Part model, mm, in its own coordinate system. Face numbers are marked on the shaded views. A direction names the side the tool comes from. Round coordinates to 2 decimals unless told otherwise and drop trailing zeros. Write each loop counter-clockwise with the first axis right and the second up, starting at its lowest first coordinate (ties: lowest second). Pieces come first, ordered by that corner, then holes. Notation, with made-up numbers: (19, 34.25) -> (37, 34.25) arc R7 ccw to (37, 38.25) -> close; hole circle Ø8 at (53, 73.5). An arc over 180 degrees is marked (long way). Use CSV: the item, a comma, the result in double quotes. Start each with the question number.
```python
from build123d import *

# Parameters (mm, degrees)
F1_DEPTH = 63.5
F2_DEPTH = 7.9375
F3_DEPTH = 25.4
F5_R     = 6.35


with BuildPart() as f1:
    # F0 (on Front) → F1 (new body, symmetric)
    with BuildSketch(Plane.XZ):
        Polygon((-41.275, 9.525), (-41.275, -9.525), (41.275, -9.525), (41.275, 9.525), (22.225, 9.525), align=None)
    extrude(amount=F1_DEPTH, both=True)

    # F0 (on Front) → F2 (join, symmetric)
    with BuildSketch(Plane.XZ):
        with BuildLine():
            add(Edge.make_bspline(
                [(-41.275, 9.525), (-40.209185, 45.154918), (21.977982, 81.660934), (57.15, 80.9752)],
                knots=[0, 0, 0, 0, 121.624881, 121.624881, 121.624881, 121.624881], degree=3))
            Line((-41.275, 9.525), (22.225, 9.525))
            Line((22.225, 9.525), (22.225, 46.0502))
            ThreePointArc((22.225, 46.0502), (32.454296, 70.745904), (57.15, 80.9752))
        make_face()
    extrude(amount=F2_DEPTH, both=True)

    # F0 (on Front) → F3 (join, symmetric)
    with BuildSketch(Plane.XZ):
        with BuildLine():
            Line((22.225, 9.525), (41.275, 9.525))
            Line((41.275, 9.525), (41.275, 46.0502))
            ThreePointArc((41.275, 46.0502), (45.92468, 57.27552), (57.15, 61.9252))
            Line((57.15, 61.9252), (60.325, 61.9252))
            Line((60.325, 61.9252), (60.325, 80.9752))
            Line((60.325, 80.9752), (57.15, 80.9752))
            ThreePointArc((57.15, 80.9752), (32.454296, 70.745904), (22.225, 46.0502))
            Line((22.225, 46.0502), (22.225, 9.525))
        make_face()
    extrude(amount=F3_DEPTH, both=True)

    # F0 (on Front) → F4 (revolve)
    with BuildSketch(Plane.XZ):
        Polygon((60.325, 85.725), (60.325, 80.9752), (85.754924, 80.9752), (85.754924, 61.9252), (60.325, 61.9252), (60.325, 57.15), (111.125, 57.15), (111.125, 85.725), align=None)
    revolve(axis=Axis((60.325, 0, 71.4375), (0, 0, -1)))

    # F5
    f5_edges = [f1.edges().sort_by_distance(p)[0] for p in [
        (41.275, -63.5, 0),
        (-41.275, -63.5, 0),
        (41.275, 63.5, 0),
        (-41.275, 63.5, 0),
    ]]
    fillet(f5_edges, radius=F5_R)


solid = f1.part
```
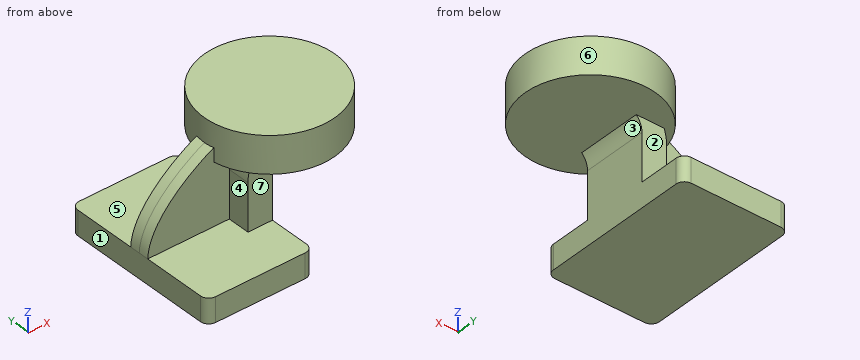
1. Band-saw the part on B-B (z = -3.5). List the corners of the cut face in (x, y) (3 decimals), then the cut area to 3 significant figures.
2. Pull direction Z, two halves, no side cores. Call the marked faces 1, 2 and 3: released by +Z, released by -Z, zero draft, split by the parting line, or undercut.
3. Drill centre lines: line 1 along Z through (x, y) = (74.5, 21) (3 decimals); line 2 along Y through (x, z) = (-19.5, 10); line 3 along Z through (x, y) = (87.5, 3) (3 decimals). Where is each one in solid material? Low to high. Write a range as [from, to].
4. Band-saw the part on D-D (y = -11). List the corners of the cut face in (x, z) (3 decimals).
5. Flat gauge pins, fed straight in: pin 1 (12 mm diameter, centred on x = 11.5, y = 44.5, fed in from +Z) (3 decimals); pin 2 (12 mm diameter, centred on x = 29, z = 29.5, fed in from +Y); pin 3 (19 mm diameter, centred on x = 32, z = 35.5, fed in from -Y). Where does each tip first touch, or does it go through?
6. Band-saw the part on C-C (x = 78). List the corners of the cut face in (y, z) (3 decimals).
7. Which spindle directions (+Z, -Z, +X, -X, +Y, -Y) get a long thin tool onto all of the face, cutting with end or side? Do the marked faces 4, 5, 6 and 7. Say none if no direction does.
8. Band-saw the part on A-A (y = 33). List the corners of the cut face in (x, z) (3 decimals), then the cut area to 3 significant figures.
Answers below:
1,outline,"(-41.275, -57.15) arc R6.35 ccw to (-34.925, -63.5) -> (34.925, -63.5) arc R6.35 ccw to (41.275, -57.15) -> (41.275, 57.15) arc R6.35 ccw to (34.925, 63.5) -> (-34.925, 63.5) arc R6.35 ccw to (-41.275, 57.15) -> close"
1,area,"10,400 mm^2"
2,face 1,"zero draft"
2,face 2,"undercut"
2,face 3,"released by -Z"
3,line 1,"z = [57.15, 61.925], [80.975, 85.725]"
3,line 2,"y = [-7.94, 7.94]"
3,line 3,"z = [57.15, 85.725]"
4,outline,"(-41.275, -9.525) -> (41.275, -9.525) -> (41.275, 46.05) arc R15.875 cw to (45.801, 57.15) -> (109.92, 57.15) -> (109.92, 85.725) -> (10.73, 85.725) -> (10.73, 57.15) -> (24.036, 57.15) arc R34.925 ccw to (22.225, 46.05) -> (22.225, 9.525) -> (-41.275, 9.525) -> close; hole (37.397, 74.853) arc R34.925 cw to (57.15, 80.975) -> (37.397, 80.975) -> close; hole (60.325, 61.925) -> (83.253, 61.925) -> (83.253, 80.975) -> (60.325, 80.975) -> close"
5,pin 1,"stops at z = 9.525"
5,pin 2,"stops at y = 25.4"
5,pin 3,"stops at y = -25.4"
6,outline,"(-47.626, 57.15) -> (47.626, 57.15) -> (47.626, 85.725) -> (-47.626, 85.725) -> close; hole (-18.283, 61.925) -> (18.283, 61.925) -> (18.283, 80.975) -> (-18.283, 80.975) -> close"
7,face 4,"-X, -Y"
7,face 5,"-X, +Y"
7,face 6,"+Z"
7,face 7,"+X, -X, -Y"
8,outline,"(-41.275, -9.525) -> (41.275, -9.525) -> (41.275, 9.525) -> (-41.275, 9.525) -> close; (21.703, 57.15) -> (98.947, 57.15) -> (98.947, 85.725) -> (21.703, 85.725) -> close"
8,area,"3,780 mm^2"
